from build123d import *

# Parameters (mm, degrees)
SKETCH1_R           = 18.4
BOSS_EXTRUDE1_DEPTH = 22
SKETCH2_R           = 17.5
BOSS_EXTRUDE2_DEPTH = 30
SKETCH3_R           = 6
BOSS_EXTRUDE4_DEPTH = 6.5
CHAMFER1_SIZE       = 1
SKETCH4_R           = 3
BOSS_EXTRUDE5_DEPTH = 3.5
BOSS_EXTRUDE6_DEPTH = 12
SKETCH6_R           = 1.7
CUT_EXTRUDE1_DEPTH  = 12


with BuildPart() as part:
    # Sketch1 → Boss-Extrude1 (new body)
    with BuildSketch(Plane.XY):
        Circle(SKETCH1_R)
    extrude(amount=BOSS_EXTRUDE1_DEPTH)

    # Sketch2 → Boss-Extrude2 (add)
    with BuildSketch(Plane(origin=(0, 0, 0), x_dir=(-1, 0, 0), z_dir=(0, 0, -1))):
        Circle(SKETCH2_R)
    extrude(amount=BOSS_EXTRUDE2_DEPTH)

    # Sketch3 → Boss-Extrude4 (add)
    with BuildSketch(Plane.XY.offset(22)):
        with Locations((7, 0)):
            Circle(SKETCH3_R)
    extrude(amount=BOSS_EXTRUDE4_DEPTH)

    # Chamfer1
    chamfer1_edges = [part.edges().sort_by_distance(p)[0] for p in [
        (1, 0, 28.5),
    ]]
    chamfer(chamfer1_edges, length=CHAMFER1_SIZE)

    # Sketch4 → Boss-Extrude5 (add)
    with BuildSketch(Plane.XY.offset(28.5)):
        with Locations((7, 0)):
            Circle(SKETCH4_R)
    extrude(amount=BOSS_EXTRUDE5_DEPTH)

    # Sketch5 → Boss-Extrude6 (add)
    with BuildSketch(Plane.XY.offset(32)):
        with BuildLine():
            ThreePointArc((10, 0), (5.658359214, 2.683281573), (5.2, -2.4))
            Line((5.2, -2.4), (8.8, -2.4))
            ThreePointArc((8.8, -2.4), (9.683281573, -1.341640786), (10, 0))
        make_face()
    extrude(amount=BOSS_EXTRUDE6_DEPTH)

    # Sketch6 → Cut-Extrude1 (cut)
    with BuildSketch(Plane.XY.offset(22)):
        with Locations((0, 15.5)):
            Circle(SKETCH6_R)
        with Locations((13.423393759, 7.75)):
            Circle(SKETCH6_R)
        with Locations((13.423393759, -7.75)):
            Circle(SKETCH6_R)
        with Locations((0, -15.5)):
            Circle(SKETCH6_R)
        with Locations((-13.423393759, -7.75)):
            Circle(SKETCH6_R)
        with Locations((-13.423393759, 7.75)):
            Circle(SKETCH6_R)
        with Locations((-15.5, 0)):
            Circle(SKETCH6_R)
        with Locations((7.75, 13.423393759)):
            Circle(SKETCH6_R)
        with Locations((7.75, -13.423393759)):
            Circle(SKETCH6_R)
    extrude(amount=-CUT_EXTRUDE1_DEPTH, mode=Mode.SUBTRACT)


solid = part.part
Model file for the job. Use its own axes, mm. A direction names the side the tool comes from. Give positions to 0.01 mm unless a question says otherwise; leave off trailing zeros. Loops run counter-clockwise (first coordinate to the right, second up) from the corner with the lowest first, then second, coordinate; pieces in that order, holes last. Notation, with made-up numbers: (0, 45) -> (17, 45) arc R21 cw to (17, 77) -> close; hole circle Ø2 at (66.25, 69.5). An arc over 180 degrees is marked (long way). Use a Markdown table: item, result. Add a question column.
(1) Tool access for faces 3 (the flat face through (8, 13, 10)), 4 (the flat face through (14.9, -9.5, 0)), 5 (the flat face through (7, -2.4, 38)): list every direction of +Z, -Z, +X, -X, +Y, -Y with a clear straight run to the whole face (end or side of a thin tool).
(2) Slice it at C-C on y = -7.75. List the corners of the cut face in (x, z).
(3) Slice it at A-A on x = 0. List the corners of the cut face in (y, z).
(4) Mould opens along X. For faces 1 (the cylindrical face through (14.208, -9.258, 16.084)), 2 (the flat face through (0, 0, 22)) say: +X half, -X half, draft (parallel to the pull), parting line (faces both ways), or undercut.
(5) Slice it at B-B on z = 21. Give the number of separate pieces and of enclosed holes in the cut face, and give its area (3 significant figures).
(6) Slice it at D-D on z = 35.5. List the corners of the cut face in (x, y), and give its area (3 significant figures).
(7) Wall check: line 1 along Y through (x, z) = (0, 15); line 2 along Y through (x, z) = (7.75, 18); line 3 along Z through (x, y) = (-11, -1.5). Give the ranges that are in metal, low to high.
(8) Drop flat-ended pins along their axis: pin 1 Ø0.7 at (x, y) = (6.5, -3) entering from +Z; pin 2 Ø4 at (x, y) = (0, 15.5) entering from +Z; pin 3 Ø1 at (x, y) = (7.5, -13.5) entering from +Z; pin 4 Ø8 at (x, y) = (12.5, 4) entering from +Z. Give the stop position or say it passes through.
Filled sheet:
| question | item | result |
|---|---|---|
| 1 | face 3 | +Z |
| 1 | face 4 | -Z |
| 1 | face 5 | +Z, +X, -X, -Y |
| 2 | outline | (-16.69, 0) -> (-15.69, 0) -> (-15.69, -30) -> (15.69, -30) -> (15.69, 0) -> (16.69, 0) -> (16.69, 22) -> (15.12, 22) -> (15.12, 10) -> (11.72, 10) -> (11.72, 22) -> (-11.72, 22) -> (-11.72, 10) -> (-15.12, 10) -> (-15.12, 22) -> (-16.69, 22) -> close |
| 3 | outline | (-18.4, 0) -> (-17.5, 0) -> (-17.5, -30) -> (17.5, -30) -> (17.5, 0) -> (18.4, 0) -> (18.4, 22) -> (17.2, 22) -> (17.2, 10) -> (13.8, 10) -> (13.8, 22) -> (-13.8, 22) -> (-13.8, 10) -> (-17.2, 10) -> (-17.2, 22) -> (-18.4, 22) -> close |
| 4 | face 1 | undercut |
| 4 | face 2 | draft |
| 5 | separate pieces | 1 |
| 5 | enclosed holes | 9 |
| 5 | area | 982 mm2 |
| 6 | outline | (5.2, -2.4) -> (8.8, -2.4) arc R3 ccw (long way) to start |
| 6 | area | 26.8 mm2 |
| 7 | line 1 | -18.4 to -17.2, -13.8 to 13.8, 17.2 to 18.4 |
| 7 | line 2 | -16.69 to -15.12, -11.72 to 11.72, 15.12 to 16.69 |
| 7 | line 3 | -30 to 22 |
| 8 | pin 1 | z = 32 |
| 8 | pin 2 | z = 22 |
| 8 | pin 3 | z = 10 |
| 8 | pin 4 | z = 44 |
